```python
from build123d import *

# Parameters (mm, degrees)
SKETCH1_W           = 42
SKETCH1_H           = 42
BOSS_EXTRUDE1_DEPTH = 48.5
SKETCH2_R           = 18
BOSS_EXTRUDE2_DEPTH = 28.5
SKETCH3_R           = 11
SKETCH3_R_2         = 4
BOSS_EXTRUDE3_DEPTH = 2
SKETCH3_2_R         = 4
BOSS_EXTRUDE4_DEPTH = 20
SKETCH4_R           = 1.5
CUT_EXTRUDE1_DEPTH  = 10
CHAMFER1_SIZE       = 5


with BuildPart() as part:
    # Sketch1 → Boss-Extrude1 (new body)
    with BuildSketch(Plane.XY):
        Rectangle(SKETCH1_W, SKETCH1_H)
    extrude(amount=BOSS_EXTRUDE1_DEPTH)

    # Sketch2 → Boss-Extrude2 (add)
    with BuildSketch(Plane.XY.offset(48.5)):
        Circle(SKETCH2_R)
    extrude(amount=BOSS_EXTRUDE2_DEPTH)

    # Sketch3 → Boss-Extrude3 (add)
    with BuildSketch(Plane.XY.offset(77)):
        Circle(SKETCH3_R)
        Circle(SKETCH3_R_2, mode=Mode.SUBTRACT)
    extrude(amount=BOSS_EXTRUDE3_DEPTH)

    # Sketch3<2> → Boss-Extrude4 (add)
    with BuildSketch(Plane.XY.offset(77)):
        Circle(SKETCH3_2_R)
    extrude(amount=BOSS_EXTRUDE4_DEPTH)

    # Sketch4 → Cut-Extrude1 (cut)
    with BuildSketch(Plane.XY.offset(77)):
        with Locations((10.606601718, -10.606601718)):
            Circle(SKETCH4_R)
        with Locations((-10.606601718, -10.606601718)):
            Circle(SKETCH4_R)
        with Locations((-10.606601718, 10.606601718)):
            Circle(SKETCH4_R)
        with Locations((10.606601718, 10.606601718)):
            Circle(SKETCH4_R)
    extrude(amount=-CUT_EXTRUDE1_DEPTH, mode=Mode.SUBTRACT)

    # Chamfer1
    chamfer1_edges = [part.edges().sort_by_distance(p)[0] for p in [
        (21, -21, 24.25),
        (-21, -21, 24.25),
        (-21, 21, 24.25),
        (21, 21, 24.25),
    ]]
    chamfer(chamfer1_edges, length=CHAMFER1_SIZE)


solid = part.part
```
Can you work these out from the model? Positions are in its coordinate system, mm. A direction names the side the tool comes from. Give positions to 0.01 mm unless a question says otherwise; leave off trailing zeros. Loops run counter-clockwise (first coordinate to the right, second up) from the corner with the lowest first, then second, coordinate; pieces in that order, holes last. Notation, with made-up numbers: M -30,-1 L 8,-1 A34 cw 8,32 Z; hole C 64.25,2.5 d3. An arc over 180 degrees is marked long. Use one line per item in the form item = value. Start each with the question number.
(1) I'm going to push flat-ended pins straight in: P1, Ø2.5, axis at x = -10.61, y = -10.61, coming from the -Z side; P2, Ø5, axis at x = 15.5, y = 1, coming from the +Z side; P3, Ø1.5, axis at x = 5, y = -9.5, coming from the +Z side; P4, Ø1.8, axis at x = 10.61, y = 10.61, coming from the +Z side. Where does each tip first touch, or does it pass through?
(2) Thinking about a two-plate mould opening in X: for faces 3 (the flat face through (21, 0, 24)), 4 (the flat face through (0, 0, 0)), 5 (the flat face through (-11, 11, 67)), which applies, released by +X, released by -X, zero draft, split by the parting line, or undercut?
(3) On a 3-axis mill with a long thin cutter (end or side, diameter ignored), from which of +Z, -Z, +X, -X, +Y, -Y can I reach the whole of each face in a straight line? I mean faces 1 (the cylindrical face through (-9.8, 11.87, 72.07)), 2 (the flat face through (0, -21, 24)). Say none if no direction works.
(4) I want a section at D-D, the plane y = 15. Write out the boundary of the cut face in (x, z), and give its area (3 significant figures).
(5) I want a section at A-A, the plane z = 39. Write out the boundary of the cut face in (x, y), and give its area (3 significant figures).
(6) I want a section at B-B, the plane y = 0. Write out the boundary of the cut face in (x, z).
(7) Please list where these lines run through material, in increasing order: line 1 (Z direction, x = -9.5, y = -7); line 2 (Z direction, x = -16, y = 17); line 3 (Y direction, x = 0.5, z = 76).
Worked out:
q1.P1 = 0
q1.P2 = 77
q1.P3 = 79
q1.P4 = 67
q2.face_3 = released by +X
q2.face_4 = zero draft
q2.face_5 = undercut
q3.face_1 = +Z
q3.face_2 = +Z, -Z, +X, -X, -Y
q4.outline = M -21,0 L 21,0 L 21,48.5 L 9.95,48.5 L 9.95,77 L -9.95,77 L -9.95,48.5 L -21,48.5 Z
q4.area = 2,600 mm²
q5.outline = M -21,-16 L -16,-21 L 16,-21 L 21,-16 L 21,16 L 16,21 L -16,21 L -21,16 Z
q5.area = 1,710 mm²
q6.outline = M -21,0 L 21,0 L 21,48.5 L 18,48.5 L 18,77 L 11,77 L 11,79 L 4,79 L 4,97 L -4,97 L -4,79 L -11,79 L -11,77 L -18,77 L -18,48.5 L -21,48.5 Z
q7.line_1 = 0 to 77
q7.line_2 = 0 to 48.5
q7.line_3 = -17.99 to 17.99
